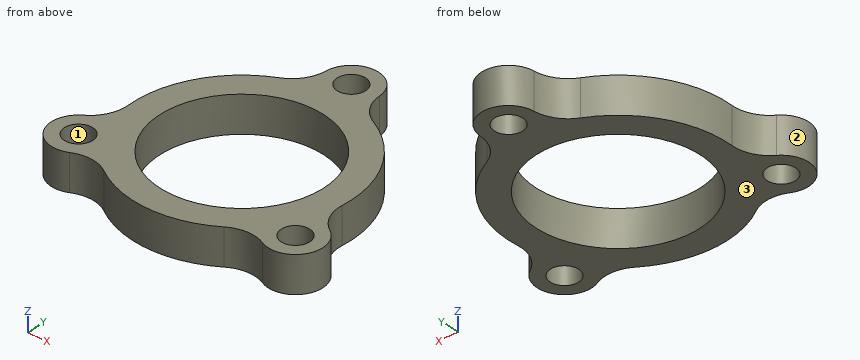
from build123d import *

# Parameters (mm, degrees)
SKETCH2_R           = 4.7625
SKETCH2_R_2         = 2.4892
SKETCH2_R_3         = 19.05
SKETCH2_R_4         = 14.2875
BOSS_EXTRUDE1_DEPTH = 6.35
FILLET2_R           = 6.35


with BuildPart() as part:
    # Sketch2 → Boss-Extrude1 (new body)
    # profile 1 of 4: a face of its own
    with BuildSketch(Plane.XY):
        with Locations((19.247414599, -11.1125)):
            Circle(SKETCH2_R)
        with Locations((19.247414599, -11.1125)):
            Circle(SKETCH2_R_2, mode=Mode.SUBTRACT)
    # profile 2 of 4: a face of its own
    with BuildSketch(Plane.XY):
        Circle(SKETCH2_R_3)
        Circle(SKETCH2_R_4, mode=Mode.SUBTRACT)
    # profile 3 of 4: a face of its own
    with BuildSketch(Plane.XY):
        with Locations((0, 22.225)):
            Circle(SKETCH2_R)
        with Locations((0, 22.225)):
            Circle(SKETCH2_R_2, mode=Mode.SUBTRACT)
    # profile 4 of 4: a face of its own
    with BuildSketch(Plane.XY):
        with Locations((-19.247414599, -11.1125)):
            Circle(SKETCH2_R)
        with Locations((-19.247414599, -11.1125)):
            Circle(SKETCH2_R_2, mode=Mode.SUBTRACT)
    extrude(amount=BOSS_EXTRUDE1_DEPTH)

    # Fillet2
    fillet2_edges = [part.edges().sort_by_distance(p)[0] for p in [
        (-17.88937524, -6.547728883, 3.175),
        (-3.27418807, 18.766517857, 3.175),
        (3.27418807, 18.766517857, 3.175),
        (17.88937524, -6.547728883, 3.175),
        (14.61518717, -12.218788974, 3.175),
        (-14.61518717, -12.218788974, 3.175),
    ]]
    fillet(fillet2_edges, radius=FILLET2_R)


solid = part.part
Part model, mm, in its own coordinate system. Face numbers are marked on the shaded views. Give positions to 0.01 mm unless a question says otherwise; leave off trailing zeros. Order: outer loops, then holes, each group sorted by start corner. A loop starts at its lowest first (then second) coordinate and runs counter-clockwise, first axis right, second up. Notation, with made-up numbers: (51.25, 73) - (108.25, 73) arc R22 cw to (108.25, 95) - close; hole circle Ø1 at (-22.75, 52). An arc over 180 degrees is marked (long way). One line per question, with ' | ' between items.
1. Pull direction Y, two halves, no side cores. Call the marked faces 1, 2 and 3: +Y half, -Y half, draft (parallel to the pull), parting line (faces both ways), or undercut.
Filled in:
face 1: undercut | face 2: parting line | face 3: draft
2. Band-saw the part on C-C on y = -12.5. List the corners of the cut face in (x, z), then the cut area to 3 significant figures.
Filled in:
outline: (-23.8, 0) - (-21.31, 0) - (-21.31, 6.35) - (-23.8, 6.35) - close; (-17.18, 0) - (-6.92, 0) - (-6.92, 6.35) - (-17.18, 6.35) - close; (6.92, 0) - (17.18, 0) - (17.18, 6.35) - (6.92, 6.35) - close; (21.31, 0) - (23.8, 0) - (23.8, 6.35) - (21.31, 6.35) - close | area: 162 mm²
3. Band-saw the part on B-B on y = 0. List the corners of the cut face in (x, z).
Filled in:
outline: (-19.05, 0) - (-14.29, 0) - (-14.29, 6.35) - (-19.05, 6.35) - close; (14.29, 0) - (19.05, 0) - (19.05, 6.35) - (14.29, 6.35) - close
4. Drop flat-ended pins along their axis: P1, Ø12, axis at x = 12.5, y = 0.5, coming from the -Z side; P2, Ø3, axis at x = 8, z = 5, coming from the +Y side; P3, Ø3, axis at x = 3, z = 5, coming from the -Y side; P4, Ø2, axis at y = -1.5, z = 5.5, coming from the +X side. Give the stop position or say it passes through.
Filled in:
P1: z = 0 | P2: y = 18.47 | P3: y = -18.99 | P4: x = 19.04
5. Drill centre lines: probe 1 along Y at (x, z) = (0, 2.25); probe 2 along X at (y, z) = (-12, 5.25); probe 3 along X at (y, z) = (-10.5, 2.25). Where is each one in solid material? Low to high.
Filled in:
probe 1: -19.05 to -14.29, 14.29 to 19.74, 24.71 to 26.99 | probe 2: -23.93 to -21.57, -16.92 to -7.75, 7.75 to 16.92, 21.57 to 23.93 | probe 3: -23.97 to -21.66, -16.83 to -9.69, 9.69 to 16.83, 21.66 to 23.97
6. Band-saw the part on A-A on x = 0. List the corners of the cut face in (y, z).
Filled in:
outline: (-19.05, 0) - (-14.29, 0) - (-14.29, 6.35) - (-19.05, 6.35) - close; (14.29, 0) - (19.74, 0) - (19.74, 6.35) - (14.29, 6.35) - close; (24.71, 0) - (26.99, 0) - (26.99, 6.35) - (24.71, 6.35) - close
7. Band-saw the part on D-D on y = 5. List the corners of the cut face in (x, z).
Filled in:
outline: (-18.38, 0) - (-13.38, 0) - (-13.38, 6.35) - (-18.38, 6.35) - close; (13.38, 0) - (18.38, 0) - (18.38, 6.35) - (13.38, 6.35) - close
